```python
from build123d import *

# Parameters (mm, degrees)
SKETCH1_R           = 1.6
BOSS_EXTRUDE1_DEPTH = 3
SKETCH3_R           = 1.6
CUT_EXTRUDE1_DEPTH  = 10


with BuildPart() as part:
    # Sketch1 → Boss-Extrude1 (new body)
    with BuildSketch(Plane(origin=(0, 0, 0), x_dir=(1, 0, 0), z_dir=(0, 1, 0))):
        Polygon((63.79786164, -35), (63.79786164, 35), (45.79786164, 35), (45.79786164, 38), (26.79786164, 38), (26.79786164, 35), (8.79786164, 35), (6.29786164, 35), (6.29786164, -35), (8.79786164, -35), (26.79786164, -35), (26.79786164, -38), (45.79786164, -38), (45.79786164, -35), align=None)
        with Locations(Location((11.79786164, -24.5, 0), (0, 0, 270))):
            Circle(SKETCH1_R, mode=Mode.SUBTRACT)
        with Locations(Location((60.29786164, -23.5, 0), (0, 0, 270))):
            Circle(SKETCH1_R, mode=Mode.SUBTRACT)
        with Locations(Location((16.29786164, 28, 0), (0, 0, 270))):
            Circle(SKETCH1_R, mode=Mode.SUBTRACT)
        with BuildLine():
            Line((45.89786164, 28), (46.668055556, 28))
            Line((46.668055556, 28), (46.668055556, 28.874884233))
            Line((46.668055556, 28.874884233), (45.637480085, 28.874884233))
            ThreePointArc((45.637480085, 28.874884233), (42.764338, 27.543595307), (45.89786164, 28))
        make_face(mode=Mode.SUBTRACT)
    extrude(amount=BOSS_EXTRUDE1_DEPTH)

    # Sketch3 → Cut-Extrude1 (cut)
    with BuildSketch(Plane.XZ):
        with Locations(Location((11.29786164, -23, 0), (0, 0, 270))):
            Circle(SKETCH3_R)
        with Locations(Location((60.79786164, -23, 0), (0, 0, 270))):
            Circle(SKETCH3_R)
        with Locations(Location((54.48786164, 32, 0), (0, 0, 270))):
            Circle(SKETCH3_R)
        with Locations(Location((28.08786164, 32, 0), (0, 0, 270))):
            Circle(SKETCH3_R)
    extrude(amount=-CUT_EXTRUDE1_DEPTH, mode=Mode.SUBTRACT)


solid = part.part
```
Check sheet for the modelled part. Datum: model origin and axes. Units: mm. A direction names the side the tool comes from. Coordinates: 2 decimals unless noted, no trailing zeros. Order: outer loops, then holes, each group sorted by start corner. A loop starts at its lowest first (then second) coordinate and runs counter-clockwise, first axis right, second up. Notation, with made-up numbers: M 35,62 L 54,62 A20 cw 54,80 Z; hole C 80,-0.5 d7. An arc over 180 degrees is marked long. One line per question, with ' | ' between items. Start each with the question number.
Item 1: Mould release check, pull along X, two halves, no side actions. Record for faces 1 (the flat face through (6.298, 1, 0)), 2 (the flat face through (45.798, 1, 37)), 3 (the cylindrical face through (58.88, 1.48, 24.24)), 4 (the flat face through (55, 1, 35)): pulls with the +X half, pulls with the -X half, needs draft (parallel to the pull), parting line crosses it, or undercut.
Item 2: Gauge pin test, flat ends, axial feed: P1, Ø0.9, axis at y = 1, z = 36, coming from the -X side; P2, Ø0.9, axis at x = 51.5, y = 2, coming from the +Z side. Record the tip position at first contact, or that the pin passes through.
Item 3: Sectioned sample at B-B on x = 44. Record the cut outline in (y, z).
Item 4: Sectioned sample at C-C on y = 2.45. Count the separate pieces of the cut face and the enclosed holes in it, and give its area (3 significant figures).
Item 5: Access from +Z, -Z, +X, -X, +Y, -Y to the whole of each face (thin tool, end or side, straight path). Record for faces 5 (the flat face through (36, 1, -38)), 6 (the cylindrical face through (42.747, 1.479, -27.605)), 7 (the flat face through (26.798, 1, 36)), 8 (the flat face through (55, 1, -35)), 9 (the flat face through (26.798, 1, -37)).
Item 6: Sectioned sample at A-A on z = -23. Record the cut outline in (x, y), and give its area (3 significant figures).
Item 7: Material ranges on line 1 (X direction, y = 1.05, z = -23); line 2 (X direction, y = 0.7, z = 32); line 3 (Z direction, x = 25.5, y = 2.55), recorded low to high.
Answer below:
1) face 1: pulls with the -X half | face 2: pulls with the +X half | face 3: undercut | face 4: needs draft
2) P1: stops at x = 26.8 | P2: stops at z = 35
3) outline: M 0,-38 L 3,-38 L 3,-29.57 L 0,-29.57 Z; M 0,-26.43 L 3,-26.43 L 3,38 L 0,38 Z
4) separate pieces: 1 | enclosed holes: 8 | area: 4,070 mm^2
5) face 5: -Z, +X, -X, +Y, -Y | face 6: +Y, -Y | face 7: +Z, -X, +Y, -Y | face 8: -Z, +X, +Y, -Y | face 9: -Z, -X, +Y, -Y
6) outline: M 6.3,0 L 9.7,0 L 9.7,3 L 6.3,3 Z; M 12.9,0 L 59.2,0 L 59.2,3 L 12.9,3 Z; M 62.4,0 L 63.8,0 L 63.8,3 L 62.4,3 Z | area: 153 mm^2
7) line 1: x = 6.3 to 9.7, 12.9 to 59.2, 62.4 to 63.8 | line 2: x = 6.3 to 26.49, 29.69 to 52.89, 56.09 to 63.8 | line 3: z = -35 to 35
